Here's how the part is built. I have some questions about the finished solid (model axes, mm). A direction names the side the tool comes from. Give positions to 0.01 mm unless a question says otherwise; leave off trailing zeros. Loops run counter-clockwise (first coordinate to the right, second up) from the corner with the lowest first, then second, coordinate; pieces in that order, holes last.
Q1. If we section it at B-B (x = 11.5): Please give me the cut outline in (y, z) (3 decimals), plus the area to 3 significant figures.
Q2. I need wall thicknesses on line 1 (X direction, y = 58, z = -116.5); line 2 (X direction, y = 11.5, z = -171); line 3 (X direction, y = 41, z = -102.5). Which ranges of each line are inside material? Lowest first, please.
Q3. We'd pull the mould along Z, two halves only. Please class faces 1 (the face through (1.049, 38.073, -176.412)), 2 (the face through (-106, 1.15, -9)), 3 (the face through (-4, 69, -163)), 4 (the face through (116.205, 0.567, -9.192)): +Z half, -Z half, draft (parallel to the pull), parting line (faces both ways), or undercut.
Q4. Will these pins go through, and if not, where does the flat tip stop? P1, Ø12, axis at x = -44.5, z = -27, coming from the +Y side; P2, Ø1, axis at x = 36, y = 60, coming from the -Z side; P3, Ø4, axis at x = -2.5, z = -8.5, coming from the +Y side; P4, Ø9.5, axis at x = -111.75, z = -9.875, coming from the -Y side.
Q5. If we section it at C-C (z = -87.5): Please give me the cut outline in (x, y), plus the area to 3 significant figures.
Q6. If we section it at A-A (x = 111): Give the number of separate pieces and of enclosed holes in the cut face, plus the area to 3 significant figures.
Q7. For faces 5 (the face through (-249, 35, -14.25)), 6 (the face through (-4, 65, -91)), 7 (the face through (-245.45, 30.48, -51.5)), 8 (the face through (208.51, 28.01, -165.4)), which set-ups out of +Z, -Z, +X, -X, +Y, -Y let a thin tool reach every point of the face, with its end or its side?
from build123d import *

# Parameters (mm, degrees)
SALIENTE_EXTRUIR1_DEPTH                              = 100
CROQUIS3_W                                           = 19.61
CROQUIS3_H                                           = 92
CROQUIS3_W_2                                         = 14.25
CORTAR_EXTRUIR2_DEPTH                                = 1047
CROQUIS4_W                                           = 21.4
CROQUIS4_H                                           = 92
CORTAR_EXTRUIR3_DEPTH                                = 1047
CROQUIS5_W                                           = 17.94
CROQUIS5_H                                           = 92
CORTAR_EXTRUIR4_DEPTH                                = 1047
CROQUIS6_W                                           = 465.66
CROQUIS6_H                                           = 136.76
CORTAR_EXTRUIR5_DEPTH                                = 65
REFRENTADO_PARA_PERNO_CON_CABEZA_HEXAGON_D           = 10.5
REFRENTADO_PARA_PERNO_CON_CABEZA_HEXAGON_DEPTH       = 90
REFRENTADO_PARA_PERNO_CON_CABEZA_HEXAGON_CBORE_D     = 13
REFRENTADO_PARA_PERNO_CON_CABEZA_HEXAGON_CBORE_DEPTH = 6.85
REFRENTADO_PARA_PERNO_CON_CABEZA_HEXAGON_TIP         = 3.15451825
CROQUIS11_R                                          = 8.5
CORTAR_EXTRUIR6_DEPTH                                = 211
CORTAR_EXTRUIR7_DEPTH                                = 528.891843468
CORTAR_EXTRUIR9_DEPTH                                = 211
REDONDEO1_R                                          = 10
REDONDEO2_R                                          = 10
REDONDEO3_R                                          = 10
REDONDEO4_R                                          = 10
CHAFL_N1_SIZE                                        = 1
REDONDEO5_R                                          = 10
SALIENTE_EXTRUIR2_START                              = 61
CROQUIS14_R                                          = 6.5
SALIENTE_EXTRUIR2_DEPTH                              = 61
CORTAR_EXTRUIR10_DEPTH                               = 550
CORTAR_EXTRUIR11_DEPTH                               = 550
CORTAR_EXTRUIR12_START                               = -550
CROQUIS18_R                                          = 8.5
CORTAR_EXTRUIR12_DEPTH                               = 550


# Some blends are built 0.0001 mm under size
with BuildPart() as part:
    # Croquis2 → Saliente-Extruir1 (new body)
    with BuildSketch(Plane(origin=(0, 0, 0), x_dir=(1, 0, 0), z_dir=(0, 1, 0))):
        Polygon((-256, 14.25), (-256, 181.28), (251, 181.28), (251, 20.92), (241, 20.92), (241, 0), (-241, 0), (-241, 14.25), align=None)
    extrude(amount=SALIENTE_EXTRUIR1_DEPTH)

    # Croquis3 → Cortar-Extruir2 (cut)
    with BuildSketch(Plane.ZY.offset(256)):
        with Locations((-171.475, 54)):
            Rectangle(CROQUIS3_W, CROQUIS3_H)
        with Locations((-7.125, 54)):
            Rectangle(CROQUIS3_W_2, CROQUIS3_H)
        Polygon((-14.25, 100), (-20.92, 100), (-22.91, 100), (-22.91, 8), (-14.25, 8), align=None)
    extrude(amount=-CORTAR_EXTRUIR2_DEPTH, mode=Mode.SUBTRACT)

    # Croquis4 → Cortar-Extruir3 (cut)
    with BuildSketch(Plane(origin=(0, 0, -161.67), x_dir=(-1, 0, 0), z_dir=(0, 0, -1))):
        with Locations((245.3, 54)):
            Rectangle(CROQUIS4_W, CROQUIS4_H)
    extrude(amount=-CORTAR_EXTRUIR3_DEPTH, mode=Mode.SUBTRACT)

    # Croquis5 → Cortar-Extruir4 (cut)
    with BuildSketch(Plane(origin=(0, 0, -161.67), x_dir=(-1, 0, 0), z_dir=(0, 0, -1))):
        with Locations((-242.03, 54)):
            Rectangle(CROQUIS5_W, CROQUIS5_H)
    extrude(amount=-CORTAR_EXTRUIR4_DEPTH, mode=Mode.SUBTRACT)

    # Croquis6 → Cortar-Extruir5 (cut)
    with BuildSketch(Plane.XZ):
        with Locations((-0.77, -92.29)):
            Rectangle(CROQUIS6_W, CROQUIS6_H)
    extrude(amount=-CORTAR_EXTRUIR5_DEPTH, mode=Mode.SUBTRACT)

    # Refrentado para perno con cabeza hexagonal de M101
    with Locations(Plane(origin=(-216, 8, -9.875), x_dir=(0, 0, 1), z_dir=(0, 1, 0))):
        with Locations((0, 0), (0, 104.25), (0, 210.25), (0, 327), (0, 427), (-46.045, 457.5), (-121.405, 457.5), (-161.53, 427), (-161.53, 327), (-161.53, 210.25), (-161.53, 104.25), (-161.53, 0)):
            CounterBoreHole(REFRENTADO_PARA_PERNO_CON_CABEZA_HEXAGON_D / 2, REFRENTADO_PARA_PERNO_CON_CABEZA_HEXAGON_CBORE_D / 2, REFRENTADO_PARA_PERNO_CON_CABEZA_HEXAGON_CBORE_DEPTH, depth=REFRENTADO_PARA_PERNO_CON_CABEZA_HEXAGON_DEPTH)
            with Locations((0, 0, -(REFRENTADO_PARA_PERNO_CON_CABEZA_HEXAGON_DEPTH + REFRENTADO_PARA_PERNO_CON_CABEZA_HEXAGON_TIP / 2))):  # 118° drill point
                Cone(0, REFRENTADO_PARA_PERNO_CON_CABEZA_HEXAGON_D / 2, REFRENTADO_PARA_PERNO_CON_CABEZA_HEXAGON_TIP, mode=Mode.SUBTRACT)

    # Croquis11 → Cortar-Extruir6 (cut)
    with BuildSketch(Plane.ZY.offset(234.6)):
        with Locations((-136.94, 22)):
            Circle(CROQUIS11_R)
        with Locations((-50.94, 22)):
            Circle(CROQUIS11_R)
    extrude(amount=-CORTAR_EXTRUIR6_DEPTH, mode=Mode.SUBTRACT)

    # Croquis12 → Cortar-Extruir7 (cut, through all)
    with BuildSketch(Plane.ZY.offset(234.6)):
        with BuildLine():
            ThreePointArc((-161.67, 69), (-141.744018282, 91.596052461), (-112.813065999, 100))
            Line((-112.813065999, 100), (-161.67, 100))
            Line((-161.67, 100), (-161.67, 69))
        make_face()
        with BuildLine():
            Line((-22.91, 100), (-71.766934001, 100))
            ThreePointArc((-71.766934001, 100), (-42.835981718, 91.596052461), (-22.91, 69))
            Line((-22.91, 69), (-22.91, 100))
        make_face()
    extrude(amount=-CORTAR_EXTRUIR7_DEPTH, mode=Mode.SUBTRACT)

    # Croquis13 → Cortar-Extruir9 (cut)
    with BuildSketch(Plane(origin=(0, 0, -161.67), x_dir=(-1, 0, 0), z_dir=(0, 0, -1))):
        with BuildLine():
            Line((-200.594633839, 100), (-233.06, 100))
            Line((-233.06, 100), (-233.06, 69))
            ThreePointArc((-233.06, 69), (-223.039009526, 91.005318547), (-200.594633839, 100))
        make_face()
        with BuildLine():
            Line((234.6, 69), (234.6, 100))
            Line((234.6, 100), (202.134633839, 100))
            ThreePointArc((202.134633839, 100), (224.579009526, 91.005318547), (234.6, 69))
        make_face()
    extrude(amount=-CORTAR_EXTRUIR9_DEPTH, mode=Mode.SUBTRACT)

    # Redondeo1
    redondeo1_edges = [part.edges().sort_by_distance(p)[0] for p in [
        (-233.6, 65, -92.29),
        (-233.6, 32.5, -160.67),
        (-233.6, 32.5, -23.91),
    ]]
    fillet(redondeo1_edges, radius=REDONDEO1_R)

    # Redondeo2
    redondeo2_edges = [part.edges().sort_by_distance(p)[0] for p in [
        (232.06, 32.5, -23.91),
    ]]
    fillet(redondeo2_edges, radius=REDONDEO2_R)

    # Redondeo3
    redondeo3_edges = [part.edges().sort_by_distance(p)[0] for p in [
        (232.06, 32.5, -160.67),
    ]]
    fillet(redondeo3_edges, radius=REDONDEO3_R)

    # Redondeo4
    # the kernel refuses this fillet: 10 mm, written as the material it adds along each edge
    with BuildSketch(Plane(origin=(-223.6, 55, -33.91), x_dir=(0, 1, 0), z_dir=(0, 0, 1))) as redondeo4_piece_1_section:
        Polygon((0, 0), (REDONDEO4_R, 0), (REDONDEO4_R, REDONDEO4_R), (0, REDONDEO4_R), align=None)
    redondeo4_piece_1 = extrude(amount=REDONDEO4_R, mode=Mode.PRIVATE)
    redondeo4_piece_1 = redondeo4_piece_1 - Plane(origin=(-223.6, 55, -33.91), x_dir=(0.7071067811865475, -0.7071067811865475, 0), z_dir=(0, 0, 1)) * Sphere(REDONDEO4_R, mode=Mode.PRIVATE)
    add(redondeo4_piece_1)
    with BuildSketch(Plane(origin=(-223.6, 55, -150.67), x_dir=(0, 1, 0), z_dir=(0, 0, -1))) as redondeo4_piece_2_section:
        Polygon((0, 0), (REDONDEO4_R, 0), (REDONDEO4_R, -REDONDEO4_R), (0, -REDONDEO4_R), align=None)
    redondeo4_piece_2 = extrude(amount=REDONDEO4_R, mode=Mode.PRIVATE)
    redondeo4_piece_2 = redondeo4_piece_2 - Plane(origin=(-223.6, 55, -150.67), x_dir=(0.7071067811865475, -0.7071067811865475, 0), z_dir=(0, 0, -1)) * Sphere(REDONDEO4_R, mode=Mode.PRIVATE)
    add(redondeo4_piece_2)
    with BuildSketch(Plane(origin=(-223.6, 65, -160.67), x_dir=(0, -1, 0), z_dir=(1, 0, 0)), Plane(origin=(222.06, 65, -23.91), x_dir=(0, -1, 0), z_dir=(-1, 0, 0))) as redondeo4_piece_3:
        with BuildLine():
            CenterArc((REDONDEO4_R, -REDONDEO4_R), REDONDEO4_R, 90, 90)
            Line((0, -REDONDEO4_R), (0, 0))
            Line((0, 0), (REDONDEO4_R, 0))
        make_face()
    extrude(amount=445.66)
    with BuildSketch(Plane(origin=(222.06, 65, -33.91), x_dir=(1, 0, 0), z_dir=(0, 0, -1))) as redondeo4_piece_4:
        with BuildLine():
            CenterArc((10 - REDONDEO4_R, REDONDEO4_R), REDONDEO4_R, 270, 90)
            Line((10 - REDONDEO4_R, 0), (10, 0))
            Line((10, 0), (10, REDONDEO4_R))
        make_face()
    revolve(axis=Axis((222.06, 65, -33.91), (0, -1, 0)), revolution_arc=90)
    with BuildSketch(Plane(origin=(232.06, 65, -150.67), x_dir=(0, -1, 0), z_dir=(0, 0, 1))) as redondeo4_piece_5:
        with BuildLine():
            CenterArc((REDONDEO4_R, -REDONDEO4_R), REDONDEO4_R, 90, 90)
            Line((0, -REDONDEO4_R), (0, 0))
            Line((0, 0), (REDONDEO4_R, 0))
        make_face()
    extrude(amount=116.76)
    with BuildSketch(Plane(origin=(222.06, 65, -150.67), x_dir=(1, 0, 0), z_dir=(0, 0, 1))) as redondeo4_piece_6:
        with BuildLine():
            CenterArc((10 - REDONDEO4_R, -REDONDEO4_R), REDONDEO4_R, 0, 90)
            Line((10 - REDONDEO4_R, 0), (10, 0))
            Line((10, 0), (10, -REDONDEO4_R))
        make_face()
    revolve(axis=Axis((222.06, 65, -150.67), (0, 1, 0)), revolution_arc=90)

    # Chaflán1
    chafl_n1_edges = [part.edges().sort_by_distance(p)[0] for p in [
        (-233.6, 22, -145.44),
        (-233.6, 22, -59.44),
    ]]
    chamfer(chafl_n1_edges, length=CHAFL_N1_SIZE - 0.0001)  # a hair under: the kernel refuses the full size

    # Redondeo5
    redondeo5_edges = [part.edges().sort_by_distance(p)[0] for p in [
        (-234.6, 38.5, -161.67),
        (-234.6, 38.5, -22.91),
        (233.06, 38.5, -22.91),
        (233.06, 38.5, -161.67),
    ]]
    fillet(redondeo5_edges, radius=REDONDEO5_R)

    # Croquis14 → Saliente-Extruir2 (add)
    with BuildSketch(Plane(origin=(0, 8, 0), x_dir=(1, 0, 0), z_dir=(0, 1, 0)).offset(SALIENTE_EXTRUIR2_START)):
        Polygon((-241, 14.25), (-241, 0), (241, 0), (241, 20.92), (251, 20.92), (251, 181.28), (-256, 181.28), (-256, 14.25), align=None)
        with Locations(Location((-216, 9.875, 0), (0, 0, 270))):
            Circle(CROQUIS14_R, mode=Mode.SUBTRACT)
        with Locations(Location((-216, 171.405, 0), (0, 0, 270))):
            Circle(CROQUIS14_R, mode=Mode.SUBTRACT)
        with Locations(Location((-111.75, 171.405, 0), (0, 0, 270))):
            Circle(CROQUIS14_R, mode=Mode.SUBTRACT)
        with Locations(Location((-5.75, 171.405, 0), (0, 0, 270))):
            Circle(CROQUIS14_R, mode=Mode.SUBTRACT)
        with Locations(Location((111, 171.405, 0), (0, 0, 270))):
            Circle(CROQUIS14_R, mode=Mode.SUBTRACT)
        with Locations(Location((211, 171.405, 0), (0, 0, 270))):
            Circle(CROQUIS14_R, mode=Mode.SUBTRACT)
        with Locations(Location((241.5, 131.28, 0), (0, 0, 270))):
            Circle(CROQUIS14_R, mode=Mode.SUBTRACT)
        with Locations(Location((241.5, 55.92, 0), (0, 0, 270))):
            Circle(CROQUIS14_R, mode=Mode.SUBTRACT)
        with Locations(Location((211, 9.875, 0), (0, 0, 270))):
            Circle(CROQUIS14_R, mode=Mode.SUBTRACT)
        with Locations(Location((111, 9.875, 0), (0, 0, 270))):
            Circle(CROQUIS14_R, mode=Mode.SUBTRACT)
        with Locations(Location((-5.75, 9.875, 0), (0, 0, 270))):
            Circle(CROQUIS14_R, mode=Mode.SUBTRACT)
        with Locations(Location((-111.75, 9.875, 0), (0, 0, 270))):
            Circle(CROQUIS14_R, mode=Mode.SUBTRACT)
        with BuildLine():
            Line((-234.6, 32.91), (-234.6, 151.67))
            ThreePointArc((-234.6, 151.67), (-231.671067812, 158.741067812), (-224.6, 161.67))
            Line((-224.6, 161.67), (223.06, 161.67))
            ThreePointArc((223.06, 161.67), (230.131067812, 158.741067812), (233.06, 151.67))
            Line((233.06, 151.67), (233.06, 32.91))
            ThreePointArc((233.06, 32.91), (230.131067812, 25.838932188), (223.06, 22.91))
            Line((223.06, 22.91), (-224.6, 22.91))
            ThreePointArc((-224.6, 22.91), (-231.671067812, 25.838932188), (-234.6, 32.91))
        make_face(mode=Mode.SUBTRACT)
    extrude(amount=-SALIENTE_EXTRUIR2_DEPTH)

    # Croquis15 → Cortar-Extruir10 (cut)
    with BuildSketch(Plane(origin=(241, 0, 0), x_dir=(0, 0, -1), z_dir=(1, 0, 0))):
        Polygon((0, 8), (10.604436087, 69), (0, 69), align=None)
    extrude(amount=-CORTAR_EXTRUIR10_DEPTH, mode=Mode.SUBTRACT)

    # Croquis16 → Cortar-Extruir11 (cut)
    with BuildSketch(Plane(origin=(251, 0, 0), x_dir=(0, 0, -1), z_dir=(1, 0, 0))):
        Polygon((171.405, 69), (181.28, 69), (181.28, 8), align=None)
    extrude(amount=-CORTAR_EXTRUIR11_DEPTH, mode=Mode.SUBTRACT)

    # Croquis18 → Cortar-Extruir12 (cut)
    with BuildSketch(Plane(origin=(-234.6, 0, 0), x_dir=(0, 0, -1), z_dir=(1, 0, 0)).offset(CORTAR_EXTRUIR12_START)):
        with Locations((136.94, 22)):
            Circle(CROQUIS18_R)
        with Locations((50.94, 22)):
            Circle(CROQUIS18_R)
    extrude(amount=CORTAR_EXTRUIR12_DEPTH, mode=Mode.SUBTRACT)


solid = part.part
Check sheet entries:
1. outline: (0, -181.28) - (8, -181.28) - (69, -171.405) - (69, -161.67) arc R54 ccw to (100, -112.813) - (100, -71.767) arc R54 ccw to (69, -22.91) - (69, -10.604) - (8, 0) - (0, 0) - (0, -23.91) - (55, -23.91) arc R10 cw to (65, -33.91) - (65, -150.67) arc R10 cw to (55, -160.67) - (0, -160.67) - close
1. area: 6,480 mm2
2. line 1: x = -256 to -233.14, 231.6 to 251
2. line 2: x = -256 to -222.49, -209.51 to -118.24, -105.26 to -12.24, 0.74 to 104.51, 117.49 to 204.51, 217.49 to 251
2. line 3: x = -256 to -233.6, 232.06 to 251
3. face 1: -Z half
3. face 2: undercut
3. face 3: draft
3. face 4: undercut
4. P1: stops at y = 83.59
4. P2: stops at z = -172.94
4. P3: stops at y = 1.15
4. P4: passes through
5. outline: (-256, 0) - (-233.6, 0) - (-233.6, 55) arc R10 cw to (-223.6, 65) - (222.06, 65) arc R10 cw to (232.06, 55) - (232.06, 0) - (251, 0) - (251, 69) - (233.06, 69) arc R32.5 ccw to (200.59, 100) - (-202.13, 100) arc R32.5 ccw to (-234.6, 69) - (-256, 69) - close
5. area: 18,800 mm2
6. separate pieces: 3
6. enclosed holes: 0
6. area: 4,980 mm2
7. face 5: +Z, -X, +Y, -Y
7. face 6: -Y
7. face 7: -X
7. face 8: +Y
